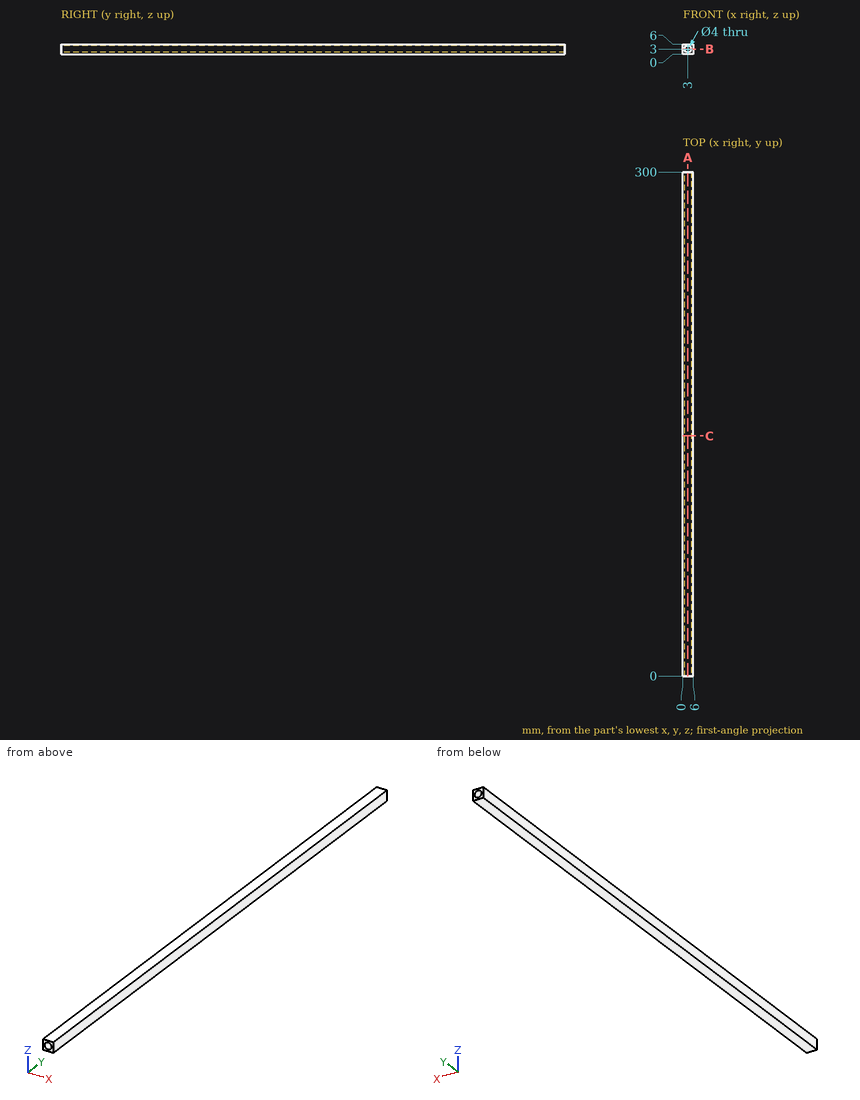
Job drawing, mm, ordinate dimensions from the low corner. One solid piece. Give positions to 0.01 mm unless a question says otherwise; leave off trailing zeros. Loops run counter-clockwise (first coordinate to the right, second up) from the corner with the lowest first, then second, coordinate; pieces in that order, holes last. Notation, with made-up numbers: (32, -33.5) - (65, -33.5) arc R19 ccw to (65, -2.5) - close; hole circle Ø8 at (30.5, -9.5). An arc over 180 degrees is marked (long way). Use one line per item in the form item = value.
(1) Cut at B-B (z = 3). Give the cut face in (x, y), then the cut area to 3 significant figures.
Determined:
outline = (0, 0) - (1, 0) - (1, 300) - (0, 300) - close; (5, 0) - (6, 0) - (6, 300) - (5, 300) - close
area = 600 mm^2
(2) Drop a flat-ended pin along its axis: P1, Ø1, axis at x = 3, z = 2, coming from the +Y side. Give the stop position or say it passes through.
Determined:
P1 = through
(3) Drill centre lines: L1, parallel to Z at x = 3, y = 77.5; L2, parallel to Z at x = 2.45, y = 177.5; L3, parallel to X at y = 131, z = 1.2. Where is each one in solid material? Low to high.
Determined:
L1 = 0 to 1, 5 to 6
L2 = 0 to 1.08, 4.92 to 6
L3 = 0 to 2.13, 3.87 to 6
(4) Cut at C-C (y = 143). Give the cut face in (x, z), then the cut area to 3 significant figures.
Determined:
outline = (0, 0) - (6, 0) - (6, 6) - (0, 6) - close; hole circle Ø4 at (3, 3)
area = 23.4 mm^2
(5) Cut at A-A (x = 3). Give the cut face in (y, z), then the cut area to 3 significant figures.
Determined:
outline = (0, 0) - (300, 0) - (300, 1) - (0, 1) - close; (0, 5) - (300, 5) - (300, 6) - (0, 6) - close
area = 600 mm^2
